Geometry: see drawing. Coordinates: mm, zero at the bounding-box minimum. A direction names the side the tool comes from. Coordinates: 2 decimals unless noted, no trailing zeros. Order: outer loops, then holes, each group sorted by start corner. A loop starts at its lowest first (then second) coordinate and runs counter-clockwise, first axis right, second up. Notation, with made-up numbers: (-38.5, 43.5) -> (5.5, 43.5) arc R15 ccw to (5.5, 47.5) -> close; hole circle Ø6 at (-7.5, 14.25). An arc over 180 degrees is marked (long way). One line per item, written item: value. Start each with the question number.
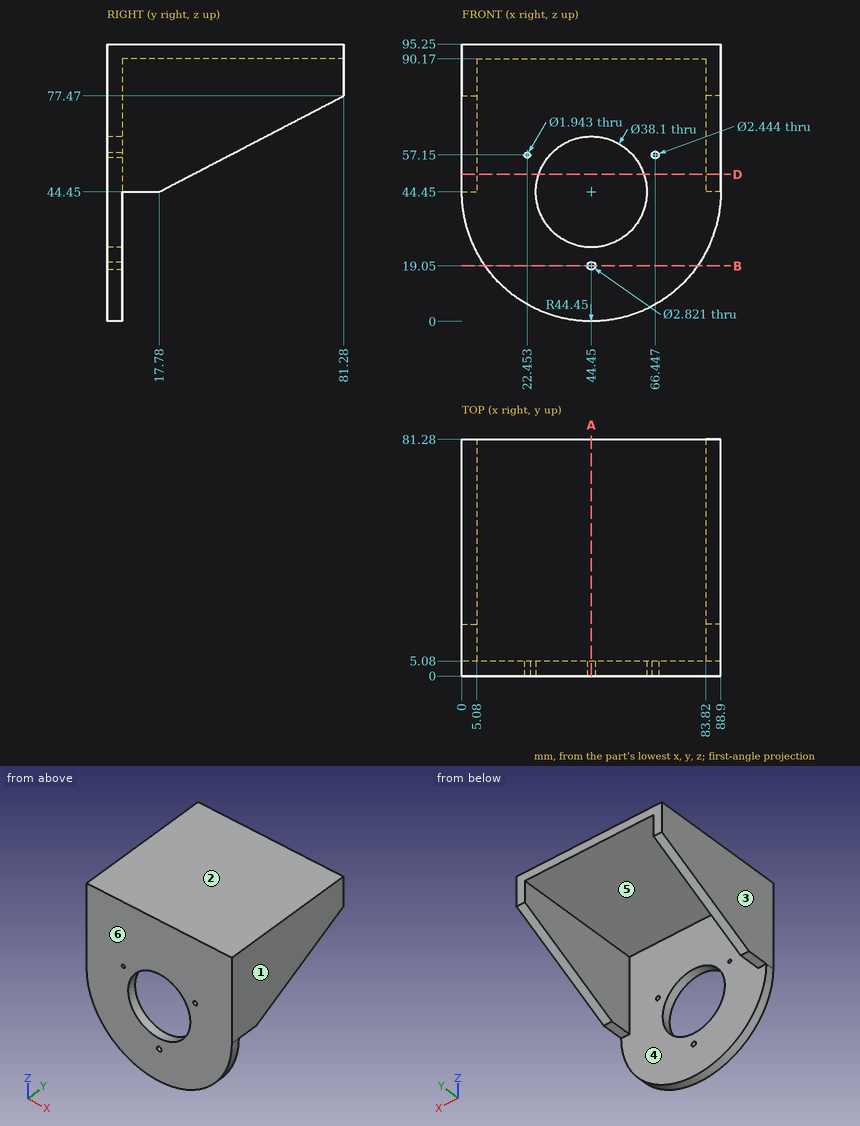
1) Section query B-B, the plane z = 19.05. Return the cut outline in (x, y), plus the area to 3 significant figures.
2) Access query for the marked faces 5 and 6. Directions: +Z, -Z, +X, -X, +Y, -Y. A direction counts if a zero-diameter tool reaches every point of the face in a straight line with its end or side. Return the directions, or none.
3) Ray query, line 1 along X through (y, z) = (58, 74.5); line 2 along X through (y, z) = (2, 57) (1 decimal); line 3 along X through (y, z) = (2.95, 44.45). Return the intervals inside material, ascending. Write a range as from..to.
4) Section query D-D, the plane z = 50.5. Return the cut outline in (x, y) (1 decimal), plus the area to 3 significant figures.
5) Section query A-A, the plane x = 44.45. Return the cut outline in (y, z).
6) Pin query (flat end, axial travel): pin 1 Ø23 at (x, y) = (62, 27.5) entering from -Z; pin 2 Ø2.5 at (x, y) = (1.5, 9) entering from -Z; pin 3 Ø1.5 at (x, z) = (30.5, 16.5) entering from +Y; pin 4 Ø1.7 at (x, z) = (44.45, 19.05) entering from -Y. Return the tip coordinate at first contact, or that it passes through.
7) Mould query, pull axis X, two halves, no side actions, for the marked faces 1, 2, 3 and 4. Classes: +X half, -X half, draft (parallel to the pull), parting line (faces both ways), or undercut.
Entries:
1. outline: (7.97, 0) -> (43.04, 0) -> (43.04, 5.08) -> (7.97, 5.08) -> close; (45.86, 0) -> (80.93, 0) -> (80.93, 5.08) -> (45.86, 5.08) -> close
1. area: 356 mm2
2. face 5: -Z, +Y
2. face 6: +Z, -Z, +X, -X, -Y
3. line 1: x = 0..5.08, 83.82..88.9
3. line 2: x = 0..21.5, 23.4..30.1, 58.8..65.2, 67.7..88.9
3. line 3: x = 0..25.4, 63.5..88.9
4. outline: (0, 0) -> (26.4, 0) -> (26.4, 5.1) -> (5.1, 5.1) -> (5.1, 29.4) -> (0, 29.4) -> close; (62.5, 0) -> (88.9, 0) -> (88.9, 29.4) -> (83.8, 29.4) -> (83.8, 5.1) -> (62.5, 5.1) -> close
4. area: 515 mm2
5. outline: (0, 0) -> (5.08, 0) -> (5.08, 17.64) -> (0, 17.64) -> close; (0, 20.46) -> (5.08, 20.46) -> (5.08, 25.4) -> (0, 25.4) -> close; (0, 63.5) -> (5.08, 63.5) -> (5.08, 90.17) -> (81.28, 90.17) -> (81.28, 95.25) -> (0, 95.25) -> close
6. pin 1: stops at z = 90.17
6. pin 2: stops at z = 44.45
6. pin 3: stops at y = 5.08
6. pin 4: passes through
7. face 1: +X half
7. face 2: draft
7. face 3: -X half
7. face 4: undercut
